Input: part model. Units: mm. Frame: model coordinates. Face numbers are marked on the shaded views. A direction names the side the tool comes from. Coordinates: 2 decimals unless noted, no trailing zeros. Write each loop counter-clockwise with the first axis right and the second up, starting at its lowest first coordinate (ties: lowest second). Pieces come first, ordered by that corner, then holes. Notation, with made-up numbers: M 32,4 L 77,4 A25 ccw 77,33 Z; hole C 78.5,16.25 d7. An arc over 180 degrees is marked long. Use one line per item in the form item = value.
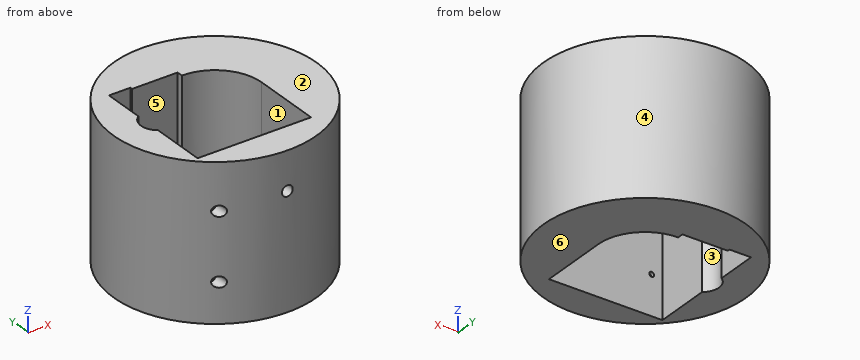
from build123d import *

# Parameters (mm, degrees)
SKETCH1_R           = 42.5
BOSS_EXTRUDE1_DEPTH = 64
SKETCH2_R           = 1
CUT_EXTRUDE1_DEPTH  = 13.5
SKETCH3_R           = 2.25
CUT_EXTRUDE2_DEPTH  = 5
SKETCH4_R           = 2.25
CUT_EXTRUDE3_DEPTH  = 12
CUT_EXTRUDE4_DEPTH  = 126.544655058


with BuildPart() as part:
    # Sketch1 → Boss-Extrude1 (new body)
    with BuildSketch(Plane(origin=(0, 0, -49.128748399), x_dir=(-1, 0, 0), z_dir=(0, 0, -1))):
        with Locations(Location((-41.816133513, 25, 0), (0, 0, 90))):
            Circle(SKETCH1_R)
        with BuildLine():
            Line((-13.801141106, 15.83484861), (-13.801141106, -4))
            Line((-13.801141106, -4), (-61.316133513, -4))
            Line((-61.316133513, -4), (-61.316133513, 25))
            ThreePointArc((-61.316133513, 25), (-55.604715746, 38.788582233), (-41.816133513, 44.5))
            Line((-41.816133513, 44.5), (-41.816133513, 47.000001781))
            Line((-41.816133513, 47.000001781), (-13.801141106, 47.000001781))
            Line((-13.801141106, 47.000001781), (-13.801141106, 34.16515139))
            Line((-13.801141106, 34.16515139), (-13.801141106, 30.744562647))
            ThreePointArc((-13.801141106, 30.744562647), (-10.801141106, 25), (-13.801141106, 19.255437353))
            Line((-13.801141106, 19.255437353), (-13.801141106, 15.83484861))
        make_face(mode=Mode.SUBTRACT)
    extrude(amount=-BOSS_EXTRUDE1_DEPTH)

    # Sketch2 → Cut-Extrude1 (cut)
    with BuildSketch(Plane(origin=(0, -17.5, 0), x_dir=(-1, 0, 0), z_dir=(0, -1, 0))):
        with Locations(Location((-18.301141106, 4.557815864, 0), (0, 0, 90))):
            Circle(SKETCH2_R)
        with Locations(Location((-18.301141106, 32.557815864, 0), (0, 0, 90))):
            Circle(SKETCH2_R)
        with Locations(Location((-41.816133513, 1.128748399, 0), (0, 0, 90))):
            Circle(SKETCH2_R)
    extrude(amount=-CUT_EXTRUDE1_DEPTH, mode=Mode.SUBTRACT)

    # Sketch3 → Cut-Extrude2 (cut)
    with BuildSketch(Plane(origin=(0, -17.5, 0), x_dir=(-1, 0, 0), z_dir=(0, -1, 0))):
        with Locations(Location((-41.816133513, 1.128748399, 0), (0, 0, 90))):
            Circle(SKETCH3_R)
        with Locations((-18.301141106, 4.557815864)):
            Circle(SKETCH3_R)
        with Locations((-18.301141106, 32.557815864)):
            Circle(SKETCH3_R)
    extrude(amount=-CUT_EXTRUDE2_DEPTH, mode=Mode.SUBTRACT)

    # Sketch4 → Cut-Extrude3 (cut)
    with BuildSketch(Plane(origin=(0, -17.5, 0), x_dir=(-1, 0, 0), z_dir=(0, -1, 0))):
        with Locations(Location((-18.301141106, 4.557815864, 0), (0, 0, 90))):
            Circle(SKETCH4_R)
        with Locations(Location((-18.301141106, 32.557815864, 0), (0, 0, 90))):
            Circle(SKETCH4_R)
    extrude(amount=-CUT_EXTRUDE3_DEPTH, mode=Mode.SUBTRACT)

    # Sketch5 → Cut-Extrude4 (cut, through all)
    with BuildSketch(Plane(origin=(0, 0, -49.128748399), x_dir=(-1, 0, 0), z_dir=(0, 0, -1))):
        Polygon((-21.801141106, 47.000001781), (-13.801141106, 47.000001781), (-13.801141106, 48.000001781), (-21.801141106, 48.000001781), (-22.748659585, 48.000001781), (-22.748659585, 47.000001781), align=None)
    extrude(amount=-CUT_EXTRUDE4_DEPTH, mode=Mode.SUBTRACT)


solid = part.part
(1) Section query C-C on x = 36.5. Return the cut outline in (y, z).
Computed:
outline = M -17.17,-49.13 L -4,-49.13 L -4,14.87 L -17.17,14.87 Z; M 47,-49.13 L 67.17,-49.13 L 67.17,14.87 L 47,14.87 Z
(2) Section query A-A on z = -9.5. Return the cut outline in (x, y), plus the area to 3 significant figures.
Computed:
outline = C 41.82,25 d85; hole M 13.8,-4 L 61.32,-4 L 61.32,25 A19.5 ccw 41.82,44.5 L 41.82,47 L 22.75,47 L 22.75,48 L 13.8,48 L 13.8,30.74 A7 ccw 13.8,19.26 Z
area = 3,350 mm^2
(3) First-contact query: pin 1 Ø7 at (x, z) = (18.5, -17) entering from -Y; pin 2 Ø4 at (y, z) = (41.5, -4) entering from +X; pin 3 Ø7 at (x, z) = (18.3, -4.56) entering from -Y; pin 4 Ø1.5 at (x, z) = (42.5, -31.5) entering from +Y. Flat tips, straight axial feed; report the tip coordinate or a pass-through.
Computed:
pin_1 = -12.6
pin_2 = 81.77
pin_3 = -12.49
pin_4 = 67.5
(4) Pull-direction query (Y, two-part tool) for the marked faces 1, 2, 3 and 4; classes: pulls with the +Y half, pulls with the -Y half, needs draft (parallel to the pull), parting line crosses it, or undercut.
Computed:
face_1 = undercut
face_2 = needs draft
face_3 = undercut
face_4 = parting line crosses it
(5) Set-up query: the marked faces 5 and 6. Return all of +Z, -Z, +X, -X, +Y, -Y with unobstructed straight access to the full face (end or side cutting, diameter ignored); none if empty.
Computed:
face_5 = +Z, -Z
face_6 = -Z, +X, -X, +Y, -Y
(6) Section query D-D on y = 50. Return the cut outline in (x, z).
Computed:
outline = M 7.45,-49.13 L 76.19,-49.13 L 76.19,14.87 L 7.45,14.87 Z
(7) Section query B-B on x = 51. Return the cut outline in (y, z).
Computed:
outline = M -16.5,-49.13 L -4,-49.13 L -4,14.87 L -16.5,14.87 Z; M 42.2,-49.13 L 66.5,-49.13 L 66.5,14.87 L 42.2,14.87 Z
(8) Line query: probe 1 along Y at (x, z) = (42.5, -9); probe 2 along Y at (x, z) = (36.5, 8.5); probe 3 along X at (y, z) = (39, 7). Output: solid intervals per line, ascending.
Computed:
probe_1 = -17.49 to -4, 44.49 to 67.49
probe_2 = -17.17 to -4, 47 to 67.17
probe_3 = 1.69 to 13.8, 55.39 to 81.94
